from build123d import *

# Parameters (mm, degrees)
BOSS_EXTRUDE1_DEPTH = 14.5
SKETCH3_R           = 1.5
CUT_EXTRUDE1_DEPTH  = 76.334255157


with BuildPart() as part:
    # Sketch2 → Boss-Extrude1 (new body)
    with BuildSketch(Plane.XY):
        with BuildLine():
            Line((0, 41.360359775), (67, 41.360359775))
            Line((67, 41.360359775), (67, 38.160359775))
            Line((67, 38.160359775), (2.044161335, 38.160359775))
            ThreePointArc((2.044161335, 38.160359775), (-1.29678146, 37.585756385), (-4.253780843, 35.927980024))
            Line((-4.253780843, 35.927980024), (-30.567780148, 14.592739527))
            ThreePointArc((-30.567780148, 14.592739527), (-33.524779531, 12.934963166), (-36.865722326, 12.360359775))
            Line((-36.865722326, 12.360359775), (-68, 12.360359775))
            Line((-68, 12.360359775), (-68, 15.560359775))
            Line((-68, 15.560359775), (-38, 15.560359775))
            ThreePointArc((-38, 15.560359775), (-34.659057205, 16.134963166), (-31.702057822, 17.792739527))
            Line((-31.702057822, 17.792739527), (-5.377247568, 39.13674548))
            ThreePointArc((-5.377247568, 39.13674548), (-3.225270493, 40.469178713), (-0.807686987, 41.218627608))
            Line((-0.807686987, 41.218627608), (0, 41.360359775))
        make_face()
    extrude(amount=BOSS_EXTRUDE1_DEPTH)

    # Sketch3 → Cut-Extrude1 (cut, through all)
    with BuildSketch(Plane(origin=(0, 41.360359775, 0), x_dir=(1, 0, 0), z_dir=(0, 1, 0))):
        with Locations(Location((6, -7.25, 0), (0, 0, 270))):
            Circle(SKETCH3_R)
        with Locations(Location((31.5, -7.25, 0), (0, 0, 270))):
            Circle(SKETCH3_R)
        with Locations(Location((57, -7.25, 0), (0, 0, 270))):
            Circle(SKETCH3_R)
        with Locations(Location((-62.214915759, -7.25, 0), (0, 0, 270))):
            Circle(SKETCH3_R)
    extrude(amount=-CUT_EXTRUDE1_DEPTH, mode=Mode.SUBTRACT)


solid = part.part
Input: part model. Units: mm. Frame: model coordinates. A direction names the side the tool comes from. Coordinates: 2 decimals unless noted, no trailing zeros. Order: outer loops, then holes, each group sorted by start corner. A loop starts at its lowest first (then second) coordinate and runs counter-clockwise, first axis right, second up. Notation, with made-up numbers: M -0.5,37 L 30.5,37 A13 ccw 30.5,57 Z; hole C -3.75,-36 d8. An arc over 180 degrees is marked long. Answer in a Markdown table with one row per item.
(1) Material intervals for line 1 (X direction, y = 40, z = 7.25); line 2 (X direction, y = 39.5, z = 7.25); line 3 (Y direction, x = 58, z = 1.5), sorted ascending. Write a range as [from, to].
Numbers:
| item | result |
|---|---|
| line 1 | x = [-4.13, 4.5], [7.5, 30], [33, 55.5], [58.5, 67] |
| line 2 | x = [-4.9, 4.5], [7.5, 30], [33, 55.5], [58.5, 67] |
| line 3 | y = [38.16, 41.36] |
(2) Section query B-B, the plane z = 7.25. Give the number of separate pieces and of enclosed holes in the cut face, plus the area to 3 significant figures.
Numbers:
| item | result |
|---|---|
| separate pieces | 5 |
| enclosed holes | 0 |
| area | 423 mm^2 |
(3) Section query D-D, the plane y = 33. Output: boundary loops of the cut face in (x, z), plus the area to 3 significant figures.
Numbers:
| item | result |
|---|---|
| outline | M -12.95,0 L -7.87,0 L -7.87,14.5 L -12.95,14.5 Z |
| area | 73.7 mm^2 |
(4) Section query C-C, the plane x = -45.5. Output: boundary loops of the cut face in (y, z), plus the area to 3 significant figures.
Numbers:
| item | result |
|---|---|
| outline | M 12.36,0 L 15.56,0 L 15.56,14.5 L 12.36,14.5 Z |
| area | 46.4 mm^2 |
(5) Access query for faces 5 (the flat face through (67, 40, 7)), 6 (the flat face through (35, 38.16, 7)). Directions: +Z, -Z, +X, -X, +Y, -Y. A direction counts if a zero-diameter tool reaches every point of the face in a straight line with its end or side. Return the directions, or none.
Numbers:
| item | result |
|---|---|
| face 5 | +Z, -Z, +X, +Y, -Y |
| face 6 | +Z, -Z, +X, -Y |
(6) Contact query for flat-ended pins moving along their axis: pin 1 Ø4.5 at (x, z) = (48, 4) entering from -Y; pin 2 Ø3 at (y, z) = (23.5, 5) entering from -X; pin 3 Ø1 at (x, z) = (-20.5, 4.5) entering from -Y. Output: stop coordinate, or through.
Numbers:
| item | result |
|---|---|
| pin 1 | stops at y = 38.16 |
| pin 2 | stops at x = -26.51 |
| pin 3 | stops at y = 22.35 |
(7) Draft query along Z for faces 1 (the cylindrical face through (-61.201, 13.983, 6.144)), 2 (the flat face through (-53, 15.56, 7)), 3 (the flat face through (-5, 36, 14.5)), 4 (the flat face through (-5, 36, 0)). Return one class per face: pulls with the +Z half, pulls with the -Z half, needs draft (parallel to the pull), parting line crosses it, or undercut.
Numbers:
| item | result |
|---|---|
| face 1 | undercut |
| face 2 | needs draft |
| face 3 | pulls with the +Z half |
| face 4 | pulls with the -Z half |
(8) Section query A-A, the plane x = 6. Output: boundary loops of the cut face in (y, z), plus the area to 3 significant figures.
Numbers:
| item | result |
|---|---|
| outline | M 38.16,0 L 41.36,0 L 41.36,5.75 L 38.16,5.75 Z; M 38.16,8.75 L 41.36,8.75 L 41.36,14.5 L 38.16,14.5 Z |
| area | 36.8 mm^2 |
